Check sheet for the modelled part. Datum: model origin and axes. Units: mm. A direction names the side the tool comes from. Give positions to 0.01 mm unless a question says otherwise; leave off trailing zeros. Loops run counter-clockwise (first coordinate to the right, second up) from the corner with the lowest first, then second, coordinate; pieces in that order, holes last. Notation, with made-up numbers: M 26,81.5 L 64,81.5 A11 cw 64,86.5 Z; hole C 78.25,22.5 d3. An arc over 180 degrees is marked long. Put each result on its own line as item: value. Start each with the question number.
```python
from build123d import *

# Parameters (mm, degrees)
SKETCH1_W          = 146.05
SKETCH1_H          = 25.4
BASE_FLANGE1_DEPTH = 1.5875
SKETCH6_R          = 3.175
CUT_EXTRUDE1_DEPTH = 2.54
CUT_EXTRUDE3_DEPTH = 2.54
SKETCH10_R         = 0.381
CUT_EXTRUDE4_DEPTH = 25.654


# Sheet-metal steps are written as plain solids
with BuildPart() as part:
    # Sketch1 → Base-Flange1 (new body)
    with BuildSketch(Plane(origin=(0, 0, 0), x_dir=(1, 0, 0), z_dir=(0, 1, 0))):
        Rectangle(SKETCH1_W, SKETCH1_H)
    extrude(amount=-BASE_FLANGE1_DEPTH)

    # Sketch6 → Cut-Extrude1 (cut)
    with BuildSketch(Plane(origin=(0, 0, 0), x_dir=(1, 0, 0), z_dir=(0, 1, 0))):
        with Locations(Location((-57.785, 0, 0), (0, 0, 270))):
            Circle(SKETCH6_R)
    extrude(amount=-CUT_EXTRUDE1_DEPTH, mode=Mode.SUBTRACT)

    # Sketch8 → Cut-Extrude3 (cut)
    with BuildSketch(Plane(origin=(0, 0, 0), x_dir=(1, 0, 0), z_dir=(0, 1, 0))):
        with BuildLine():
            Line((43.7515, 1.5875), (46.556638938, 1.5875))
            ThreePointArc((46.556638938, 1.5875), (52.705, 6.35), (58.853361062, 1.5875))
            Line((58.853361062, 1.5875), (61.6585, 1.5875))
            ThreePointArc((61.6585, 1.5875), (63.246, 0), (61.6585, -1.5875))
            Line((61.6585, -1.5875), (58.853361062, -1.5875))
            ThreePointArc((58.853361062, -1.5875), (52.705, -6.35), (46.556638938, -1.5875))
            Line((46.556638938, -1.5875), (43.7515, -1.5875))
            ThreePointArc((43.7515, -1.5875), (42.164, 0), (43.7515, 1.5875))
        make_face()
    extrude(amount=-CUT_EXTRUDE3_DEPTH, mode=Mode.SUBTRACT)

    # Sketch10 → Cut-Extrude4 (cut)
    with BuildSketch(Plane.XY.offset(12.7)):
        with Locations((-25.398772406, 0)):
            Circle(SKETCH10_R)
    extrude(amount=-CUT_EXTRUDE4_DEPTH, mode=Mode.SUBTRACT)


solid = part.part
```
Q1. Access from +Z, -Z, +X, -X, +Y, -Y to the whole of each face (thin tool, end or side, straight path). Record for faces 1 (the face through (-50, 0, 0)), 2 (the face through (52.82, -0.78, 6.35)).
Q2. Mould release check, pull along Z, two halves, no side actions. Record for faces 3 (the face through (23, 0, 0)), 4 (the face through (-54.637, -0.783, -0.413)): pulls with the +Z half, pulls with the -Z half, needs draft (parallel to the pull), parting line crosses it, or undercut.
Q3. Thickness scan on line 1 along X through (y, z) = (-0.55, 0) (3 decimals); line 2 along Z through (x, y) = (45.5, -1); line 3 along X through (y, z) = (-1.45, -1.75) (3 decimals). Record the ranges inside material, lowest first. Write a range as [from, to].
Q4. Section check A-A, the plane z = 0. Record the cut outline in (x, y) (1 decimal), then the cut area to 3 significant figures.
Q5. Section check C-C, the plane x = 57.5. Record the cut outline in (y, z).
Q6. Section check B-B, the plane y = -1.1. Give the number of separate pieces and of enclosed holes in the cut face, then the cut area to 3 significant figures.
Found:
1. face 1: +Z, -Z, +X, -X, +Y
1. face 2: +Y, -Y
2. face 3: needs draft
2. face 4: undercut
3. line 1: x = [-73.025, -60.96], [-54.61, 42.164], [63.246, 73.025]
3. line 2: z = [-12.7, -1.59], [1.59, 12.7]
3. line 3: x = [-73.025, -60.434], [-55.136, 46.601], [58.809, 73.025]
4. outline: M -73,-1.6 L -61,-1.6 L -61,0 L -73,0 Z; M -54.6,-1.6 L 42.2,-1.6 L 42.2,0 L -25,0 A0.4 cw -25.8,0 L -54.6,0 Z; M 63.2,-1.6 L 73,-1.6 L 73,0 L 63.2,0 Z
4. area: 188 mm^2
5. outline: M -1.59,-12.7 L 0,-12.7 L 0,-4.16 L -1.59,-4.16 Z; M -1.59,4.16 L 0,4.16 L 0,12.7 L -1.59,12.7 Z
6. separate pieces: 1
6. enclosed holes: 2
6. area: 3,530 mm^2
